```python
from build123d import *

# Parameters (mm, degrees)
F0_R     = 3.302
F0_W     = 52
F0_H     = 52
F0_R_2   = 1.9128263044
F0_R_3   = 17
F1_DEPTH = 12.7
F2_DEPTH = 25.4
F3_R     = 6.35


with BuildPart() as f1:
    # F0 (on Front) → F1 (new body)
    with BuildSketch(Plane.XZ):
        with BuildLine():
            Line((108.4265169831, 0.0004552842), (32.2265169831, 152.4004552842))
            Line((32.2265169831, 152.4004552842), (-107.4734830169, 152.4004552842))
            Line((-107.4734830169, 152.4004552842), (-107.4734830169, -76.1995447158))
            add(Edge.make_bspline(
                [(-84.2229677556, -114.2995447158), (-85.0358593396, -95.7832909802), (-85.4194185281, -76.1871889735), (-107.4734830169, -76.1995447158)],
                knots=[0, 0, 0, 0, 44.6340280494, 44.6340280494, 44.6340280494, 44.6340280494], degree=3))
            Line((-84.2229677556, -114.2995447158), (108.4265169831, -114.2995447158))
            Line((108.4265169831, -114.2995447158), (108.4265169831, 0.0004552842))
        make_face()
        with Locations((-88.4234830169, -57.1371889735)):
            Circle(F0_R, mode=Mode.SUBTRACT)
        with Locations((-88.4234830169, -19.0371889735)):
            Circle(F0_R, mode=Mode.SUBTRACT)
        with Locations((-69.4084768891, 38.0714893565)):
            Rectangle(F0_W, F0_H, mode=Mode.SUBTRACT)
        with Locations((-88.4234830169, 95.2504552842)):
            Circle(F0_R, mode=Mode.SUBTRACT)
        with Locations((-88.4234830169, 133.3504552842)):
            Circle(F0_R, mode=Mode.SUBTRACT)
        with Locations((-69.4084768891, 38.0714893565)):
            Rectangle(F0_W, F0_H)
        with Locations((-90.4046768891, 17.0752893565)):
            Circle(F0_R_2, mode=Mode.SUBTRACT)
        with Locations((-48.4122768891, 17.0752893565)):
            Circle(F0_R_2, mode=Mode.SUBTRACT)
        with Locations((-69.4084763527, 38.0714898929)):
            Circle(F0_R_3, mode=Mode.SUBTRACT)
        with Locations((-90.4046768891, 59.0676893565)):
            Circle(F0_R_2, mode=Mode.SUBTRACT)
        with Locations((-48.4122768891, 59.0676893565)):
            Circle(F0_R_2, mode=Mode.SUBTRACT)
    extrude(amount=F1_DEPTH)

    # F0 (on Front) → F2 (cut)
    with BuildSketch(Plane.XZ):
        with BuildLine():
            Line((108.4265169831, 0.0004552842), (32.2265169831, 152.4004552842))
            Line((32.2265169831, 152.4004552842), (-107.4734830169, 152.4004552842))
            Line((-107.4734830169, 152.4004552842), (-107.4734830169, -76.1995447158))
            add(Edge.make_bspline(
                [(-84.2229677556, -114.2995447158), (-85.0358593396, -95.7832909802), (-85.4194185281, -76.1871889735), (-107.4734830169, -76.1995447158)],
                knots=[0, 0, 0, 0, 44.6340280494, 44.6340280494, 44.6340280494, 44.6340280494], degree=3))
            Line((-84.2229677556, -114.2995447158), (108.4265169831, -114.2995447158))
            Line((108.4265169831, -114.2995447158), (108.4265169831, 0.0004552842))
        make_face()
        with Locations((-88.4234830169, -57.1371889735)):
            Circle(F0_R, mode=Mode.SUBTRACT)
        with Locations((-88.4234830169, -19.0371889735)):
            Circle(F0_R, mode=Mode.SUBTRACT)
        with Locations((-69.4084768891, 38.0714893565)):
            Rectangle(F0_W, F0_H, mode=Mode.SUBTRACT)
        with Locations((-88.4234830169, 95.2504552842)):
            Circle(F0_R, mode=Mode.SUBTRACT)
        with Locations((-88.4234830169, 133.3504552842)):
            Circle(F0_R, mode=Mode.SUBTRACT)
    extrude(amount=-F2_DEPTH, mode=Mode.SUBTRACT)

    # F3
    f3_edges = [f1.edges().sort_by_distance(p)[0] for p in [
        (-107.473483, -6.35, 152.400455),
        (-107.473483, -6.35, -76.199545),
        (108.426517, -6.35, 0.000455),
        (32.226517, -6.35, 152.400455),
    ]]
    fillet(f3_edges, radius=F3_R)


solid = f1.part
```
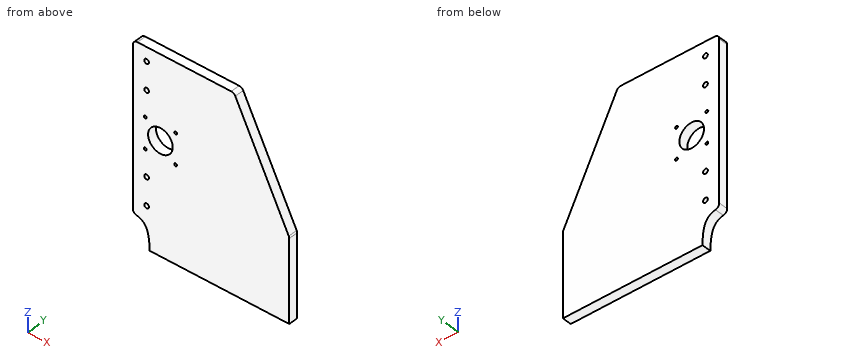
Input: part model. Units: mm. Frame: model coordinates. Give positions to 0.01 mm unless a question says otherwise; leave off trailing zeros. Order: outer loops, then holes, each group sorted by start corner. A loop starts at its lowest first (then second) coordinate and runs counter-clockwise, first axis right, second up. Notation, with made-up numbers: (30, -39.75) -> (69, -39.75) arc R22 ccw to (69, -31.75) -> close; hole circle Ø5 at (-26, 84.5). An arc over 180 degrees is marked (long way). Write each question's results on one line, items separated by ' | '. Start each with the question number.
Item 1: Cut plane C-C on x = 89.5. Return the cut outline in (y, z).
Item 2: Cut plane B-B on z = 112.5. Return the cut outline in (x, y), then the cut area to 3 significant figures.
Item 3: Cut plane A-A on x = -62. Return the cut outline in (y, z), then the cut area to 3 significant figures.
Item 4: Contact query for flat-ended pins moving along their axis: P1, Ø2, axis at x = 53, y = -6.5, coming from the +Z side; P2, Ø4, axis at x = 13, z = 8.5, coming from the +Y side; P3, Ø3, axis at x = -90.4, z = 17.08, coming from the +Y side; P4, Ø3, axis at x = 50, y = -5.5, coming from the +Z side. Output: stop coordinate, or through.
Item 5: Line query: line 1 (Z direction, x = -59, y = -7.25); line 2 (Z direction, x = -67, y = -11); line 3 (X direction, y = -11, z = -91.5). Output: solid intervals per line, ascending.
Item 6: Cut plane D-D on y = -2.75. Give the number of separate pieces and of enclosed holes in the cut face, then the cut area to 3 significant figures.
Established:
1) outline: (-12.7, -114.3) -> (0, -114.3) -> (0, 37.85) -> (-12.7, 37.85) -> close
2) outline: (-107.47, -12.7) -> (52.18, -12.7) -> (52.18, 0) -> (-107.47, 0) -> close | area: 2,030 mm^2
3) outline: (-12.7, -114.3) -> (0, -114.3) -> (0, 22.77) -> (-12.7, 22.77) -> close; (-12.7, 53.37) -> (0, 53.37) -> (0, 152.4) -> (-12.7, 152.4) -> close | area: 3,000 mm^2
4) P1: z = 112.85 | P2: y = 0 | P3: through | P4: z = 119.85
5) line 1: -114.3 to 24.63, 51.51 to 152.4 | line 2: -114.3 to 21.24, 54.9 to 152.4 | line 3: -86.78 to 108.43
6) separate pieces: 1 | enclosed holes: 9 | area: 49,900 mm^2
